Geometry check sheet. Reference: the model listing, model coordinates, mm. A direction names the side the tool comes from. Round coordinates to 2 decimals unless told otherwise and drop trailing zeros. Write each loop counter-clockwise with the first axis right and the second up, starting at its lowest first coordinate (ties: lowest second). Pieces come first, ordered by that corner, then holes. Notation, with made-up numbers: (69, 28.5) - (127, 28.5) arc R30 cw to (127, 56.5) - close; hole circle Ø8 at (-40, -36). An arc over 180 degrees is marked (long way). Return JSON: item names as keys, results as strings.
```python
from build123d import *

# Parameters (mm, degrees)
SKETCH1_W           = 530.8
SKETCH1_H           = 170.8
SKETCH1_R           = 2.5
BOSS_EXTRUDE1_DEPTH = 10


with BuildPart() as part:
    # Sketch1 → Boss-Extrude1 (new body)
    with BuildSketch(Plane(origin=(0, 0, 0), x_dir=(1, 0, 0), z_dir=(0, 1, 0))):
        with Locations((223.844914973, 70.363620549)):
            Rectangle(SKETCH1_W, SKETCH1_H)
        with Locations(Location((-8.655085027, 17.863620549, 0), (0, 0, 270))):
            Circle(SKETCH1_R, mode=Mode.SUBTRACT)
        with Locations(Location((96.344914973, 17.863620549, 0), (0, 0, 90))):
            Circle(SKETCH1_R, mode=Mode.SUBTRACT)
        with Locations(Location((96.344914973, 122.863620549, 0), (0, 0, 270))):
            Circle(SKETCH1_R, mode=Mode.SUBTRACT)
        with Locations(Location((-8.655085027, 122.863620549, 0), (0, 0, 90))):
            Circle(SKETCH1_R, mode=Mode.SUBTRACT)
        with Locations(Location((111.344914973, 17.863620549, 0), (0, 0, 270))):
            Circle(SKETCH1_R, mode=Mode.SUBTRACT)
        with Locations(Location((216.344914973, 17.863620549, 0), (0, 0, 90))):
            Circle(SKETCH1_R, mode=Mode.SUBTRACT)
        with Locations(Location((111.344914973, 122.863620549, 0), (0, 0, 90))):
            Circle(SKETCH1_R, mode=Mode.SUBTRACT)
        with Locations(Location((216.344914973, 122.863620549, 0), (0, 0, 270))):
            Circle(SKETCH1_R, mode=Mode.SUBTRACT)
        with Locations(Location((231.344914973, 17.863620549, 0), (0, 0, 270))):
            Circle(SKETCH1_R, mode=Mode.SUBTRACT)
        with Locations(Location((336.344914973, 17.863620549, 0), (0, 0, 90))):
            Circle(SKETCH1_R, mode=Mode.SUBTRACT)
        with Locations(Location((231.344914973, 122.863620549, 0), (0, 0, 90))):
            Circle(SKETCH1_R, mode=Mode.SUBTRACT)
        with Locations(Location((336.344914973, 122.863620549, 0), (0, 0, 270))):
            Circle(SKETCH1_R, mode=Mode.SUBTRACT)
        with Locations(Location((351.344914973, 17.863620549, 0), (0, 0, 270))):
            Circle(SKETCH1_R, mode=Mode.SUBTRACT)
        with Locations(Location((456.344914973, 17.863620549, 0), (0, 0, 90))):
            Circle(SKETCH1_R, mode=Mode.SUBTRACT)
        with Locations(Location((351.344914973, 122.863620549, 0), (0, 0, 90))):
            Circle(SKETCH1_R, mode=Mode.SUBTRACT)
        with Locations(Location((456.344914973, 122.863620549, 0), (0, 0, 270))):
            Circle(SKETCH1_R, mode=Mode.SUBTRACT)
        with Locations(Location((9.244914973, 149.413620549, 0), (0, 0, 270))):
            Circle(SKETCH1_R, mode=Mode.SUBTRACT)
        with Locations(Location((95.084914973, 149.413620549, 0), (0, 0, 270))):
            Circle(SKETCH1_R, mode=Mode.SUBTRACT)
        with Locations(Location((180.924914973, 149.413620549, 0), (0, 0, 270))):
            Circle(SKETCH1_R, mode=Mode.SUBTRACT)
        with Locations(Location((266.764914973, 149.413620549, 0), (0, 0, 270))):
            Circle(SKETCH1_R, mode=Mode.SUBTRACT)
        with Locations(Location((352.604914973, 149.413620549, 0), (0, 0, 270))):
            Circle(SKETCH1_R, mode=Mode.SUBTRACT)
        with Locations(Location((438.444914973, 149.413620549, 0), (0, 0, 270))):
            Circle(SKETCH1_R, mode=Mode.SUBTRACT)
        with Locations(Location((480.384698099, 35.763620549, 0), (0, 0, 270))):
            Circle(SKETCH1_R, mode=Mode.SUBTRACT)
        with Locations(Location((438.444914973, -8.686379451, 0), (0, 0, 90))):
            Circle(SKETCH1_R, mode=Mode.SUBTRACT)
        with Locations(Location((352.604914973, -8.686379451, 0), (0, 0, 90))):
            Circle(SKETCH1_R, mode=Mode.SUBTRACT)
        with Locations(Location((266.764914973, -8.686379451, 0), (0, 0, 90))):
            Circle(SKETCH1_R, mode=Mode.SUBTRACT)
        with Locations(Location((180.924914973, -8.686379451, 0), (0, 0, 90))):
            Circle(SKETCH1_R, mode=Mode.SUBTRACT)
        with Locations(Location((95.084914973, -8.686379451, 0), (0, 0, 90))):
            Circle(SKETCH1_R, mode=Mode.SUBTRACT)
        with Locations(Location((9.244914973, -8.686379451, 0), (0, 0, 90))):
            Circle(SKETCH1_R, mode=Mode.SUBTRACT)
        with Locations(Location((480.384698099, 104.963620549, 0), (0, 0, 270))):
            Circle(SKETCH1_R, mode=Mode.SUBTRACT)
        with Locations(Location((-32.694868153, 35.763620549, 0), (0, 0, 90))):
            Circle(SKETCH1_R, mode=Mode.SUBTRACT)
        with Locations(Location((-32.694868153, 104.963620549, 0), (0, 0, 90))):
            Circle(SKETCH1_R, mode=Mode.SUBTRACT)
        with BuildLine():
            Line((146.344914973, 130.363620549), (181.344914973, 130.363620549))
            ThreePointArc((181.344914973, 130.363620549), (208.039088797, 114.557794374), (223.844914973, 87.863620549))
            ThreePointArc((223.844914973, 87.863620549), (239.650741149, 114.557794374), (266.344914973, 130.363620549))
            Line((266.344914973, 130.363620549), (301.344914973, 130.363620549))
            ThreePointArc((301.344914973, 130.363620549), (328.039088797, 114.557794374), (343.844914973, 87.863620549))
            ThreePointArc((343.844914973, 87.863620549), (359.650741149, 114.557794374), (386.344914973, 130.363620549))
            Line((386.344914973, 130.363620549), (421.344914973, 130.363620549))
            ThreePointArc((421.344914973, 130.363620549), (448.039088797, 114.557794374), (463.844914973, 87.863620549))
            Line((463.844914973, 87.863620549), (463.844914973, 52.863620549))
            ThreePointArc((463.844914973, 52.863620549), (448.039088797, 26.169446725), (421.344914973, 10.363620549))
            Line((421.344914973, 10.363620549), (386.344914973, 10.363620549))
            ThreePointArc((386.344914973, 10.363620549), (359.650741149, 26.169446725), (343.844914973, 52.863620549))
            ThreePointArc((343.844914973, 52.863620549), (328.039088797, 26.169446725), (301.344914973, 10.363620549))
            Line((301.344914973, 10.363620549), (266.344914973, 10.363620549))
            ThreePointArc((266.344914973, 10.363620549), (239.650741149, 26.169446725), (223.844914973, 52.863620549))
            ThreePointArc((223.844914973, 52.863620549), (208.039088797, 26.169446725), (181.344914973, 10.363620549))
            Line((181.344914973, 10.363620549), (146.344914973, 10.363620549))
            ThreePointArc((146.344914973, 10.363620549), (119.650741149, 26.169446725), (103.844914973, 52.863620549))
            ThreePointArc((103.844914973, 52.863620549), (88.039088797, 26.169446725), (61.344914973, 10.363620549))
            Line((61.344914973, 10.363620549), (26.344914973, 10.363620549))
            ThreePointArc((26.344914973, 10.363620549), (-0.349258851, 26.169446725), (-16.155085027, 52.863620549))
            Line((-16.155085027, 52.863620549), (-16.155085027, 87.863620549))
            ThreePointArc((-16.155085027, 87.863620549), (-0.349258851, 114.557794374), (26.344914973, 130.363620549))
            Line((26.344914973, 130.363620549), (61.344914973, 130.363620549))
            ThreePointArc((61.344914973, 130.363620549), (88.039088797, 114.557794374), (103.844914973, 87.863620549))
            ThreePointArc((103.844914973, 87.863620549), (119.650741149, 114.557794374), (146.344914973, 130.363620549))
        make_face(mode=Mode.SUBTRACT)
    extrude(amount=BOSS_EXTRUDE1_DEPTH)


solid = part.part
```
(1) Gauge pin test, flat end, axial feed: pin 1 (4.5 mm diameter, centred on x = 438.44, z = 8.69, fed in from +Y). Record the tip position at first contact, or that the pin passes through.
Response values:
{"pin 1": "passes through"}
(2) Section check B-B, the plane x = 322. Enter the section's corners in (y, z).
Response values:
{"outline": "(0, -155.76) - (10, -155.76) - (10, -119.87) - (0, -119.87) - close; (0, -20.86) - (10, -20.86) - (10, 15.04) - (0, 15.04) - close"}
(3) Release check for a two-part mould opening along Z. For faces 3 (the face through (-16.155, 5, -70)), 4 (the face through (220, 5, 15.036)), 5 (the face through (489.245, 5, -69)) record: pulls with the +Z half, pulls with the -Z half, needs draft (parallel to the pull), parting line crosses it, or undercut.
Response values:
{"face 3": "undercut", "face 4": "pulls with the +Z half", "face 5": "needs draft"}
(4) Material ranges on line 1 along X through (y, z) = (6, -52.5); line 2 along X through (y, z) = (2.75, -63); line 3 along Z through (x, y) = (354.5, 9.5), recorded low to high. Write a range as [from, to].
Response values:
{"line 1": "x = [-41.56, -16.05], [103.74, 103.95], [223.74, 223.95], [343.74, 343.95], [463.74, 489.24]", "line 2": "x = [-41.56, -16.16], [463.84, 489.24]", "line 3": "z = [-155.76, -151.04], [-147.78, -108.72], [-32.01, 7.06], [10.32, 15.04]"}
(5) Section check A-A, the plane z = -73. Enter the section's corners in (x, y).
Response values:
{"outline": "(-41.56, 0) - (-16.16, 0) - (-16.16, 10) - (-41.56, 10) - close; (463.84, 0) - (489.24, 0) - (489.24, 10) - (463.84, 10) - close"}
(6) Section check C-C, the plane z = -48. Enter the section's corners in (x, y), plus the area to 3 significant figures.
Response values:
{"outline": "(-41.56, 0) - (-14.52, 0) - (-14.52, 10) - (-41.56, 10) - close; (102.21, 0) - (105.48, 0) - (105.48, 10) - (102.21, 10) - close; (222.21, 0) - (225.48, 0) - (225.48, 10) - (222.21, 10) - close; (342.21, 0) - (345.48, 0) - (345.48, 10) - (342.21, 10) - close; (462.21, 0) - (489.24, 0) - (489.24, 10) - (462.21, 10) - close", "area": "639 mm^2"}
(7) Section check D-D, the plane y = 1.75. Give the number of separate pieces and of enclosed holes in the cut face, plus the area to 3 significant figures.
Response values:
{"separate pieces": "1", "enclosed holes": "33", "area": "41,900 mm^2"}
(8) Access from +Z, -Z, +X, -X, +Y, -Y to the whole of each face (thin tool, end or side, straight path). Record for faces 1 (the face through (119.96, 4.93, -25.86)), 2 (the face through (220, 0, -110)).
Response values:
{"face 1": "+Y, -Y", "face 2": "+Z, -Z, +X, -X, -Y"}
